For this review, take the finished solid that the model builds, in its own axes (mm). A direction names the side the tool comes from. Round coordinates to 2 decimals unless told otherwise and drop trailing zeros. Write each loop counter-clockwise with the first axis right and the second up, starting at its lowest first coordinate (ties: lowest second). Pieces come first, ordered by that corner, then holes. Notation, with made-up numbers: (-25.5, 26.5) -> (19.5, 26.5) arc R28 cw to (19.5, 54.5) -> close; hole circle Ø1 at (27, 16.5). An arc over 180 degrees is marked (long way). Answer in a Markdown table with one row per item. Add a question column.
```python
from build123d import *

# Parameters (mm, degrees)
SKETCH1_W                                      = 10.5
SKETCH1_H                                      = 8.5
EXTRUDE1_DEPTH                                 = 4.75
SKETCH3_W                                      = 9.75
SKETCH3_H                                      = 8.5
EXTRUDE4_DEPTH                                 = 2
SKETCH4_W                                      = 9.4
SKETCH4_H                                      = 7.8
EXTRUDE5_DEPTH                                 = 0.75
SKETCH5_W                                      = 4
SKETCH5_H                                      = 2.75
EXTRUDE6_DEPTH                                 = 3.75
CBORE_FOR_0_SOCKET_HEAD_CAP_SCREW1_D           = 1.778
CBORE_FOR_0_SOCKET_HEAD_CAP_SCREW1_CBORE_D     = 3.175
CBORE_FOR_0_SOCKET_HEAD_CAP_SCREW1_CBORE_DEPTH = 1.524
FILLET1_R                                      = 1


with BuildPart() as part:
    # Sketch1 → Extrude1 (new body)
    with BuildSketch(Plane(origin=(0, 0, 0), x_dir=(1, 0, 0), z_dir=(0, 1, 0))):
        Rectangle(SKETCH1_W, SKETCH1_H)
    extrude(amount=EXTRUDE1_DEPTH)

    # Sketch3 → Extrude4 (cut)
    with BuildSketch(Plane(origin=(0, 4.75, 0), x_dir=(1, 0, 0), z_dir=(0, 1, 0))):
        with Locations((-0.375, 0)):
            Rectangle(SKETCH3_W, SKETCH3_H)
    extrude(amount=-EXTRUDE4_DEPTH, mode=Mode.SUBTRACT)

    # Sketch4 → Extrude5 (cut)
    with BuildSketch(Plane(origin=(0, 2.75, 0), x_dir=(1, 0, 0), z_dir=(0, 1, 0))):
        with Locations((-0.2, 0)):
            Rectangle(SKETCH4_W, SKETCH4_H)
    extrude(amount=-EXTRUDE5_DEPTH, mode=Mode.SUBTRACT)

    # Sketch5 → Extrude6 (add)
    with BuildSketch(Plane.XY.offset(4.25)):
        with Locations((1.25, 1.375)):
            Rectangle(SKETCH5_W, SKETCH5_H)
    extrude(amount=EXTRUDE6_DEPTH)

    # CBORE for #0 Socket Head Cap Screw1 (through all)
    with Locations(Plane(origin=(1.25, 0, 6), x_dir=(0, 0, -1), z_dir=(0, -1, 0))):
        with Locations((0, 0)):
            CounterBoreHole(CBORE_FOR_0_SOCKET_HEAD_CAP_SCREW1_D / 2, CBORE_FOR_0_SOCKET_HEAD_CAP_SCREW1_CBORE_D / 2, CBORE_FOR_0_SOCKET_HEAD_CAP_SCREW1_CBORE_DEPTH)

    # Fillet1
    # the kernel refuses this fillet: 1 mm, written as the material it adds along each edge
    with BuildSketch(Plane(origin=(3.25, 2.75, 4.25), x_dir=(0, 0, 1), z_dir=(0, -1, 0))) as fillet1_piece_1:
        with BuildLine():
            CenterArc((FILLET1_R, -FILLET1_R), FILLET1_R, 90, 90)
            Line((0, -FILLET1_R), (0, 0))
            Line((0, 0), (FILLET1_R, 0))
        make_face()
    extrude(amount=2.75)
    with BuildSketch(Plane(origin=(-0.75, 0, 4.25), x_dir=(-1, 0, 0), z_dir=(0, 1, 0))) as fillet1_piece_2:
        with BuildLine():
            CenterArc((FILLET1_R, FILLET1_R), FILLET1_R, 180, 90)
            Line((0, FILLET1_R), (0, 0))
            Line((0, 0), (FILLET1_R, 0))
        make_face()
    extrude(amount=2.75)
    with BuildSketch(Plane(origin=(4.5, 2.75, -3.9), x_dir=(0, 0, 1), z_dir=(0, -1, 0)), Plane(origin=(-4.9, 2.75, -3.9), x_dir=(1, 0, 0), z_dir=(0, -1, 0)), Plane(origin=(-4.9, 2.75, 3.9), x_dir=(0, 0, -1), z_dir=(0, -1, 0))) as fillet1_piece_3:
        with BuildLine():
            CenterArc((FILLET1_R, FILLET1_R), FILLET1_R, 180, 90)
            Line((0, FILLET1_R), (0, 0))
            Line((0, 0), (FILLET1_R, 0))
        make_face()
    extrude(amount=0.75)
    with BuildSketch(Plane(origin=(4.5, 2.75, 3.9), x_dir=(0, 0, -1), z_dir=(0, -1, 0))) as fillet1_piece_4:
        with BuildLine():
            CenterArc((FILLET1_R, -FILLET1_R), FILLET1_R, 90, 90)
            Line((0, -FILLET1_R), (0, 0))
            Line((0, 0), (FILLET1_R, 0))
        make_face()
    extrude(amount=0.75)
    # the kernel refuses this fillet: 1 mm, written as the material it takes off along each edge
    with BuildSketch(Plane(origin=(5.25, -2.5, -4.25), x_dir=(-1, 0, 0), z_dir=(0, 1, 0)), Plane(origin=(5.25, -2.5, 4.25), x_dir=(0, 0, -1), z_dir=(0, 1, 0))) as fillet1_2_piece_1:
        with BuildLine():
            CenterArc((FILLET1_R, FILLET1_R), FILLET1_R, 180, 90)
            Line((0, FILLET1_R), (0, 0))
            Line((0, 0), (FILLET1_R, 0))
        make_face()
    extrude(amount=9.75, mode=Mode.SUBTRACT)
    with BuildSketch(Plane(origin=(3.25, 5.25, 8), x_dir=(0, 0, -1), z_dir=(0, -1, 0))) as fillet1_2_piece_2:
        with BuildLine():
            CenterArc((FILLET1_R, -FILLET1_R), FILLET1_R, 90, 90)
            Line((0, -FILLET1_R), (0, 0))
            Line((0, 0), (FILLET1_R, 0))
        make_face()
    extrude(amount=7.75, mode=Mode.SUBTRACT)
    with BuildSketch(Plane(origin=(-0.75, -2.5, 8), x_dir=(1, 0, 0), z_dir=(0, 1, 0)), Plane(origin=(-5.25, -2.5, -4.25), x_dir=(0, 0, 1), z_dir=(0, 1, 0)), Plane(origin=(-5.25, -2.5, 4.25), x_dir=(1, 0, 0), z_dir=(0, 1, 0))) as fillet1_2_piece_3:
        with BuildLine():
            CenterArc((FILLET1_R, FILLET1_R), FILLET1_R, 180, 90)
            Line((0, FILLET1_R), (0, 0))
            Line((0, 0), (FILLET1_R, 0))
        make_face()
    extrude(amount=7.75, mode=Mode.SUBTRACT)


solid = part.part
```
1. For L1, parallel to X at y = 2.25, z = 6; L2, parallel to X at y = 0.3, z = 6; L3, parallel to X at y = 3.45, z = -1.75, list the stretches that pass through material, from the lowest coordinate up. Write a range as [from, to].
2. We need section B-B (z = 6). Write out the cut boundary in (x, y).
3. Tool access review of faces 4 (the cylindrical face through (-4.599, 2.38, 3.615)), 5 (the cylindrical face through (-4.949, 1.356, -3.965)), 6 (the flat face through (-3, 1, 4.25)), 7 (the flat face through (1.27, 1.524, 4.96)): name each direction out of +Z, -Z, +X, -X, +Y, -Y from which nothing blocks a thin tool from reaching the whole face with its end or side.
4. Clearance check with flat-ended pins moving along their axes: pin 1 Ø2.5 at (x, z) = (-1.5, -0.5) entering from +Y; pin 2 Ø1.9 at (y, z) = (1.5, 6) entering from +X; pin 3 Ø1.4 at (y, z) = (1.5, 6) entering from -X. State where each tip first meets the part, or that it passes through.
5. We need section D-D (z = -1.5). Write out the cut boundary in (x, y), plus the area to 3 significant figures.
6. We need section A-A (x = 1.25). Write out the cut boundary in (y, z), plus the area to 3 significant figures.
7. The part is to be moulded in two halves that separate along X. For faces 1 (the cylindrical face through (1.517, 2.146, 6.848)), 2 (the flat face through (0, 1, -4.25)), 3 (the flat face through (3.25, 1, 6)), say which applies: pulls with the +X half, pulls with the -X half, needs draft (parallel to the pull), parting line crosses it, or undercut.
Response:
| question | item | result |
|---|---|---|
| 1 | L1 | [-0.75, 0.36], [2.14, 3.25] |
| 1 | L2 | [-0.75, -0.34], [2.84, 3.25] |
| 1 | L3 | [4.5, 5.25] |
| 2 | outline | (-0.75, 0) -> (-0.34, 0) -> (-0.34, 1.52) -> (0.36, 1.52) -> (0.36, 2.75) -> (-0.75, 2.75) -> close; (2.14, 1.52) -> (2.84, 1.52) -> (2.84, 0) -> (3.25, 0) -> (3.25, 2.75) -> (2.14, 2.75) -> close |
| 3 | face 4 | +Y |
| 3 | face 5 | -Z, -X, +Y, -Y |
| 3 | face 6 | +Z, -X, +Y, -Y |
| 3 | face 7 | -Y |
| 4 | pin 1 | y = 2 |
| 4 | pin 2 | x = 3.27 |
| 4 | pin 3 | x = -0.75 |
| 5 | outline | (-5.25, 0) -> (5.25, 0) -> (5.25, 4.75) -> (4.5, 4.75) -> (4.5, 2) -> (-4.9, 2) -> (-4.9, 2.75) -> (-5.25, 2.75) -> close |
| 5 | area | 23.3 mm2 |
| 6 | outline | (0, -4.25) -> (2.75, -4.25) -> (2.75, -3.9) -> (2, -3.9) -> (2, 3.9) -> (2.75, 3.9) -> (2.75, 5.11) -> (1.52, 5.11) -> (1.52, 4.41) -> (0, 4.41) -> close; (0, 7.59) -> (1.52, 7.59) -> (1.52, 6.89) -> (2.75, 6.89) -> (2.75, 8) -> (0, 8) -> close |
| 6 | area | 20.8 mm2 |
| 7 | face 1 | undercut |
| 7 | face 2 | needs draft |
| 7 | face 3 | pulls with the +X half |
